from build123d import *

# Parameters (mm, degrees)
FILLET1_R           = 2
FILLET2_R           = 6
SCALE1_SCALE        = 0.85
SKETCH4_R           = 10.6
CUT_EXTRUDE2_DEPTH  = 51.23590774
SKETCH9_R           = 2.25
BOSS_EXTRUDE1_DEPTH = 4.25
FILLET4_R           = 3


with BuildPart() as part:
    # Sketch2 → Revolve1 (revolve)
    with BuildSketch(Plane(origin=(0, 0, 0), x_dir=(0, 0, -1), z_dir=(1, 0, 0))):
        Polygon((10.1, 0), (10.1, 6.971067812), (62.23, 59.101067812), (75, 59.101067812), (75, 54.101067812), (64.301067812, 54.101067812), (15.1, 4.9), (20, 0), align=None)
    revolve(axis=Axis((0, 0, 0), (0, 1, 0)))

    # Fillet1
    fillet1_edges = [part.edges().sort_by_distance(p)[0] for p in [
        (0, 4.9, 15.1),
    ]]
    fillet(fillet1_edges, radius=FILLET1_R)

    # Fillet2
    fillet2_edges = [part.edges().sort_by_distance(p)[0] for p in [
        (0, 6.971067812, 10.1),
    ]]
    fillet(fillet2_edges, radius=FILLET2_R)


with BuildPart() as part_1:
    # Scale1: scaled about (0, 40.216103787, 0)
    add(part.part.scale(SCALE1_SCALE).moved(Location((0, 6.032415568, 0))))

    # Sketch4 → Cut-Extrude2 (cut, through all)
    with BuildSketch(Plane.XZ.offset(-6.032415568)):
        Circle(SKETCH4_R)
    extrude(amount=-CUT_EXTRUDE2_DEPTH, mode=Mode.SUBTRACT)

    # Sketch9 → Boss-Extrude1 (add)
    with BuildSketch(Plane.XZ.offset(-52.018323208)):
        with BuildLine():
            Line((-62.154465971, 14.492663996), (-63.814937276, -0.932057036))
            ThreePointArc((-63.814937276, -0.932057036), (-64.336549414, 0.385954164), (-65.60066074, 1.027246064))
            Line((-65.60066074, 1.027246064), (-70.240082919, 1.526679887))
            ThreePointArc((-70.240082919, 1.526679887), (-75.563426885, 8.134403325), (-68.955703447, 13.45774729))
            Line((-68.955703447, 13.45774729), (-64.316281268, 12.958313466))
            ThreePointArc((-64.316281268, 12.958313466), (-62.944644221, 13.315867039), (-62.154465971, 14.492663996))
        make_face()
        with Locations((-69.597893183, 7.492213588)):
            Circle(SKETCH9_R, mode=Mode.SUBTRACT)
        with BuildLine():
            Line((-0.932057036, 63.814937276), (14.492663996, 62.154465971))
            ThreePointArc((14.492663996, 62.154465971), (13.315867039, 62.944644221), (12.958313466, 64.316281268))
            Line((12.958313466, 64.316281268), (13.45774729, 68.955703447))
            ThreePointArc((13.45774729, 68.955703447), (8.134403325, 75.563426885), (1.526679887, 70.240082919))
            Line((1.526679887, 70.240082919), (1.027246064, 65.60066074))
            ThreePointArc((1.027246064, 65.60066074), (0.385954164, 64.336549414), (-0.932057036, 63.814937276))
        make_face()
        with Locations((7.492213588, 69.597893183)):
            Circle(SKETCH9_R, mode=Mode.SUBTRACT)
        with BuildLine():
            Line((63.814937276, 0.932057036), (62.154465971, -14.492663996))
            ThreePointArc((62.154465971, -14.492663996), (62.944644221, -13.315867039), (64.316281268, -12.958313466))
            Line((64.316281268, -12.958313466), (68.955703447, -13.45774729))
            ThreePointArc((68.955703447, -13.45774729), (75.563426885, -8.134403325), (70.240082919, -1.526679887))
            Line((70.240082919, -1.526679887), (65.60066074, -1.027246064))
            ThreePointArc((65.60066074, -1.027246064), (64.336549414, -0.385954164), (63.814937276, 0.932057036))
        make_face()
        with Locations((69.597893183, -7.492213588)):
            Circle(SKETCH9_R, mode=Mode.SUBTRACT)
        with BuildLine():
            Line((-14.492663996, -62.154465971), (0.932057036, -63.814937276))
            ThreePointArc((0.932057036, -63.814937276), (-0.385954164, -64.336549414), (-1.027246064, -65.60066074))
            Line((-1.027246064, -65.60066074), (-1.526679887, -70.240082919))
            ThreePointArc((-1.526679887, -70.240082919), (-8.134403325, -75.563426885), (-13.45774729, -68.955703447))
            Line((-13.45774729, -68.955703447), (-12.958313466, -64.316281268))
            ThreePointArc((-12.958313466, -64.316281268), (-13.315867039, -62.944644221), (-14.492663996, -62.154465971))
        make_face()
        with Locations((-7.492213588, -69.597893183)):
            Circle(SKETCH9_R, mode=Mode.SUBTRACT)
    extrude(amount=-BOSS_EXTRUDE1_DEPTH)

    # Fillet4
    fillet4_edges = [part_1.edges().sort_by_distance(p)[0] for p in [
        (-7.495331881, 13.972823208, 7.495331881),
        (0, 52.018323208, 54.65590764),
    ]]
    fillet(fillet4_edges, radius=FILLET4_R)


solid = part_1.part
Geometry: final body of the model. Coordinates: model frame, mm. A direction names the side the tool comes from. Give positions to 0.01 mm unless a question says otherwise; leave off trailing zeros. Write each loop counter-clockwise with the first axis right and the second up, starting at its lowest first coordinate (ties: lowest second). Pieces come first, ordered by that corner, then holes. Notation, with made-up numbers: (75.5, -30) -> (96.5, -30) arc R26 cw to (96.5, -3) -> close; hole circle Ø6 at (60, -23). An arc over 180 degrees is marked (long way). Answer as a JSON object with one key per item and string values.
1. Ray query, probe 1 along X at (y, z) = (37, 22.5); probe 2 along X at (y, z) = (9.5, 0); probe 3 along Y at (x, z) = (-1.5, -60.5). Return the intervals inside material, ascending. Write a range as from..to.
Ans:
{"probe 1": "x = -32.63..-24.99, 24.99..32.63", "probe 2": "x = -13.69..-10.6, 10.6..13.69", "probe 3": "y = 52.02..56.27"}
2. Cut plane A-A on y = 42.5. Output: boundary loops of the cut face in (x, z), and give its area (3 significant figures).
Ans:
{"outline": "circle Ø90.28 at (0, 0); hole circle Ø78.25 at (0, 0)", "area": "1,590 mm^2"}
3. Mould query, pull axis Z, two halves, no side actions, for faces 1 (the flat face through (67.95, 54.11, -1.28)), 2 (the flat face through (-67.888, 54.114, 1.273)), 3 (the cylindrical face through (-71.846, 54.114, 7.591)). Classes: pulls with the +Z half, pulls with the -Z half, needs draft (parallel to the pull), parting line crosses it, or undercut.
Ans:
{"face 1": "pulls with the +Z half", "face 2": "pulls with the -Z half", "face 3": "undercut"}
4. Access query for faces 4 (the flat face through (66.604, 54.114, -13.205)), 5 (the flat face through (11, 6.032, 0)), 6 (the flat face through (6, 52.018, -56)). Directions: +Z, -Z, +X, -X, +Y, -Y. A direction counts if a zero-diameter tool reaches every point of the face in a straight line with its end or side. Return the directions, or none.
Ans:
{"face 4": "-Z, +Y, -Y", "face 5": "+Z, -Z, +X, -X, -Y", "face 6": "-Y"}
5. Contact query for flat-ended pins moving along their axis: pin 1 (2.5 mm diameter, centred on x = -7.49, z = -69.6, fed in from +Y); pin 2 (1 mm diameter, centred on x = -10.5, z = -15, fed in from +Y); pin 3 (1 mm diameter, centred on x = -4.5, z = -27.5, fed in from -Y); pin 4 (5 mm diameter, centred on x = 10.5, z = -41, fed in from -Y). Output: stop coordinate, or through.
Ans:
{"pin 1": "passes through", "pin 2": "stops at y = 22.18", "pin 3": "stops at y = 24.73", "pin 4": "stops at y = 37.19"}
